Part model, mm, in its own coordinate system. Face numbers are marked on the shaded views. Round coordinates to 2 decimals unless told otherwise and drop trailing zeros. Order: outer loops, then holes, each group sorted by start corner. A loop starts at its lowest first (then second) coordinate and runs counter-clockwise, first axis right, second up. Notation, with made-up numbers: (19.5, 81) - (25.5, 81) arc R20 cw to (25.5, 107) - close; hole circle Ø1 at (-26, 23). An arc over 180 degrees is marked (long way). Return JSON: item names as keys, results as strings. Group by question number.
Item 1: Drop flat-ended pins along their axis: pin 1 (1.2 mm diameter, centred on x = -1.5, y = 2, fed in from -Z); pin 2 (2 mm diameter, centred on x = -3.5, z = 11, fed in from -Y); pin 3 (1.5 mm diameter, centred on y = 1.5, z = 5, fed in from -X); pin 4 (2.5 mm diameter, centred on x = -7.78, z = 7.78, fed in from +Y). Give the stop position or say it passes through.
Item 2: Probe probe 1 along Z at (x, y) = (3.5, 1.8); probe 2 along Y at (x, z) = (11.5, -0.5); probe 3 along X at (y, z) = (2.2, 10.5). List the from-to ranges inside material, lowest first.
Item 3: Saw through at D-D on y = -0.5. List the corners of the cut face in (x, z) (3 decimals).
Item 4: Saw through at A-A on y = 1.9. List the corners of the cut face in (x, z), and give its area (3 significant figures).
Item 5: Saw through at C-C on x = 0. List the corners of the cut face in (y, z) (3 decimals).
Item 6: Saw through at B-B on z = 0. List the corners of the cut face in (x, y).
Item 7: Two-plate mould, pull along Y, no slides. Class the marked faces 1 and 2: released by +Y, released by -Y, zero draft, split by the parting line, or undercut.
```python
from build123d import *

# Parameters (mm, degrees)
SKETCH_1_R      = 15
SKETCH_1_R_2    = 1.3
EXTRUDE_2_DEPTH = 1
SKETCH_2_W      = 5.5
SKETCH_2_H      = 5.5
SKETCH_2_W_2    = 10.16
SKETCH_2_H_2    = 3.68
EXTRUDE_5_DEPTH = 1.5
SKETCH_3_W      = 5
SKETCH_3_H      = 3.37
EXTRUDE_7_DEPTH = 1.5


with BuildPart() as part:
    # 草图1 → 凸台-拉伸2 (new body)
    with BuildSketch(Plane(origin=(0, 0, 0), x_dir=(1, 0, 0), z_dir=(0, 1, 0))):
        Circle(SKETCH_1_R)
        with Locations((-7.778174593, 7.778174593)):
            Circle(SKETCH_1_R_2, mode=Mode.SUBTRACT)
        with Locations((7.778174593, 7.778174593)):
            Circle(SKETCH_1_R_2, mode=Mode.SUBTRACT)
        with Locations((7.778174593, -7.778174593)):
            Circle(SKETCH_1_R_2, mode=Mode.SUBTRACT)
        with Locations((-7.778174593, -7.778174593)):
            Circle(SKETCH_1_R_2, mode=Mode.SUBTRACT)
    extrude(amount=EXTRUDE_2_DEPTH)

    # 草图2 → 凸台-拉伸5 (add)
    with BuildSketch(Plane(origin=(0, 1, 0), x_dir=(1, 0, 0), z_dir=(0, 1, 0))):
        Rectangle(SKETCH_2_W, SKETCH_2_H)
        with Locations((-1.15, -9.46)):
            Rectangle(SKETCH_2_W_2, SKETCH_2_H_2)
    extrude(amount=EXTRUDE_5_DEPTH)

    # 草图3 → 凸台-拉伸7 (add)
    with BuildSketch(Plane.XZ):
        Rectangle(SKETCH_3_W, SKETCH_3_H)
    extrude(amount=EXTRUDE_7_DEPTH)


solid = part.part
```
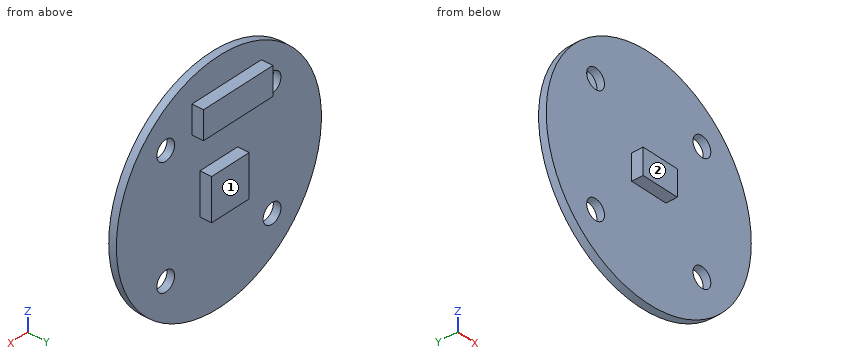
Filled in:
{
 "1": {"pin 1": "stops at z = -2.75", "pin 2": "stops at y = 0", "pin 3": "stops at x = -14.33", "pin 4": "passes through"},
 "2": {"probe 1": "z = 7.62 to 11.3", "probe 2": "y = 0 to 1", "probe 3": "x = -6.23 to 3.93"},
 "3": {"outline": "(-2.5, -1.685) - (2.5, -1.685) - (2.5, 1.685) - (-2.5, 1.685) - close"},
 "4": {"outline": "(-6.23, 7.62) - (3.93, 7.62) - (3.93, 11.3) - (-6.23, 11.3) - close; (-2.75, -2.75) - (2.75, -2.75) - (2.75, 2.75) - (-2.75, 2.75) - close", "area": "67.6 mm^2"},
 "5": {"outline": "(-1.5, -1.685) - (0, -1.685) - (0, -15) - (1, -15) - (1, -2.75) - (2.5, -2.75) - (2.5, 2.75) - (1, 2.75) - (1, 7.62) - (2.5, 7.62) - (2.5, 11.3) - (1, 11.3) - (1, 15) - (0, 15) - (0, 1.685) - (-1.5, 1.685) - close"},
 "6": {"outline": "(-15, 0) - (-2.5, 0) - (-2.5, -1.5) - (2.5, -1.5) - (2.5, 0) - (15, 0) - (15, 1) - (2.75, 1) - (2.75, 2.5) - (-2.75, 2.5) - (-2.75, 1) - (-15, 1) - close"},
 "7": {"face 1": "released by +Y", "face 2": "released by -Y"}
}
